```python
from build123d import *

# Parameters (mm, degrees)
F0_W     = 254
F0_H     = 323.85
F1_DEPTH = 6.35
F3_DEPTH = 12.7


with BuildPart() as f1:
    # F0 (on Right) → F1 (new body, symmetric)
    with BuildSketch(Plane.YZ):
        Rectangle(F0_W, F0_H)
    extrude(amount=F1_DEPTH, both=True)

    # F2 (on Right) → F3 (cut, symmetric)
    with BuildSketch(Plane.YZ):
        Polygon((0, 75.19789), (0, 7.023266), (47.736385, 75.19789), align=None)
        with BuildLine():
            Line((-47.736385, 75.19789), (0, 7.023266))
            Line((0, 7.023266), (0, 75.19789))
            Line((0, 75.19789), (0, 108.623266))
            ThreePointArc((0, 108.623266), (-40.580881, 115.77877), (-47.736385, 75.19789))
        make_face()
        with BuildLine():
            Line((0, 75.19789), (47.736385, 75.19789))
            ThreePointArc((47.736385, 75.19789), (40.580881, 115.77877), (0, 108.623266))
            Line((0, 108.623266), (0, 75.19789))
        make_face()
    extrude(amount=F3_DEPTH, both=True, mode=Mode.SUBTRACT)


solid = f1.part
```
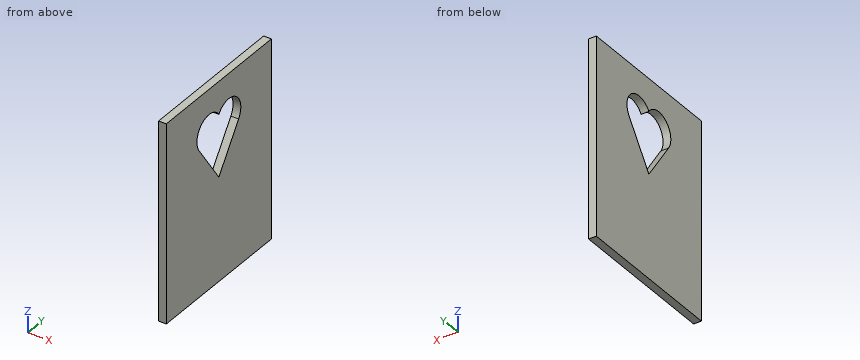
Model file for the job. Use its own axes, mm. Coordinates: 2 decimals unless noted, no trailing zeros. Write each loop counter-clockwise with the first axis right and the second up, starting at its lowest first coordinate (ties: lowest second). Pieces come first, ordered by that corner, then holes. Notation, with made-up numbers: (-13, 8.5) - (12, 8.5) arc R12 cw to (12, 12.5) - close; hole circle Ø1 at (18, 64.5). An arc over 180 degrees is marked (long way). Use a Markdown table: item, result. Add a question column.
Item 1: Band-saw the part on A-A, the plane y = 5. Write the cut outline in (x, z) (3 decimals), and give its area (3 significant figures).
Item 2: Drill centre lines: line 1 along Y through (x, z) = (-0.5, 109); line 2 along Y through (x, z) = (-5, 36.5); line 3 along Z through (x, y) = (-1.25, -27) (3 decimals). Where is each one in solid material? Low to high.
Item 3: Band-saw the part on C-C, the plane x = -3.5. Write the cut outline in (y, z) (3 decimals), and give its area (3 significant figures).
Item 4: Band-saw the part on B-B, the plane z = 31. Write the cut outline in (x, y).
A:
| question | item | result |
|---|---|---|
| 1 | outline | (-6.35, -161.925) - (6.35, -161.925) - (6.35, 14.164) - (-6.35, 14.164) - close; (-6.35, 114.114) - (6.35, 114.114) - (6.35, 161.925) - (-6.35, 161.925) - close |
| 1 | area | 2,840 mm² |
| 2 | line 1 | y = -127 to -47.47, -0.27 to 0.27, 47.47 to 127 |
| 2 | line 2 | y = -127 to -20.64, 20.64 to 127 |
| 2 | line 3 | z = -161.925 to 45.583, 120.879 to 161.925 |
| 3 | outline | (-127, -161.925) - (127, -161.925) - (127, 161.925) - (-127, 161.925) - close; hole (-47.736, 75.198) - (0, 7.023) - (47.736, 75.198) arc R29.138 ccw to (0, 108.623) arc R29.138 ccw to start |
| 3 | area | 74,700 mm² |
| 4 | outline | (-6.35, -127) - (6.35, -127) - (6.35, -16.79) - (-6.35, -16.79) - close; (-6.35, 16.79) - (6.35, 16.79) - (6.35, 127) - (-6.35, 127) - close |
